Solid Edge part; units mm, degrees
sketch "Sketch1" plane through (0, 0, 0) normal (0, 0, 1) x (1, 0, 0)
  line L0 (-12, 10) -> (12, 10)
  line L1 (12, -10) -> (12, 10)
  line L2 (-12, -10) -> (12, -10)
  line L3 (-12, -10) -> (-12, 10)
  circle A0 centre (-7, 5) radius 2.2
  circle A1 centre (-7, -5) radius 2.2
  circle A2 centre (7, -5) radius 2.2
  circle A3 centre (7, 5) radius 2.2
extrude "Protrusion1" add sketch "Sketch1" against normal blind 6
Geometry: final body of the model. Coordinates: model frame, mm. Give positions to 0.01 mm unless a question says otherwise; leave off trailing zeros. Write each loop counter-clockwise with the first axis right and the second up, starting at its lowest first coordinate (ties: lowest second). Pieces come first, ordered by that corner, then holes.
1. Section query C-C, the plane z = -0.9. Return loops of the section in (x, y).
2. Draft query along Y for faces 1 (the cylindrical face through (-4.9, 5.66, -2.96)), 2 (the flat face through (0, 10, -3)), 3 (the flat face through (0, -10, -3)), 4 (the flat face through (12, 0, -3)). Return one class per face: released by +Y, released by -Y, zero draft, split by the parting line, or undercut.
3. Section query A-A, the plane y = -5. Return loops of the section in (x, z), then the cut area to 3 significant figures.
4. Section query B-B, the plane x = -7. Return loops of the section in (y, z), then the cut area to 3 significant figures.
5. Pin query (flat end, axial travel): P1, Ø5.5, axis at x = -7, y = 5, coming from the -Z side. Return the tip coordinate at first contact, or that it passes through.
6. Line query: probe 1 along Y at (x, z) = (7, -1.4); probe 2 along X at (y, z) = (-6.5, -1.75); probe 3 along X at (y, z) = (-3.75, -4.85). Output: solid intervals per line, ascending.
Computed:
1. outline: (-12, -10) - (12, -10) - (12, 10) - (-12, 10) - close; hole circle Ø4.4 at (-7, -5); hole circle Ø4.4 at (-7, 5); hole circle Ø4.4 at (7, -5); hole circle Ø4.4 at (7, 5)
2. face 1: undercut
2. face 2: released by +Y
2. face 3: released by -Y
2. face 4: zero draft
3. outline: (-12, -6) - (-9.2, -6) - (-9.2, 0) - (-12, 0) - close; (-4.8, -6) - (4.8, -6) - (4.8, 0) - (-4.8, 0) - close; (9.2, -6) - (12, -6) - (12, 0) - (9.2, 0) - close
3. area: 91.2 mm2
4. outline: (-10, -6) - (-7.2, -6) - (-7.2, 0) - (-10, 0) - close; (-2.8, -6) - (2.8, -6) - (2.8, 0) - (-2.8, 0) - close; (7.2, -6) - (10, -6) - (10, 0) - (7.2, 0) - close
4. area: 67.2 mm2
5. P1: stops at z = -6
6. probe 1: y = -10 to -7.2, -2.8 to 2.8, 7.2 to 10
6. probe 2: x = -12 to -8.61, -5.39 to 5.39, 8.61 to 12
6. probe 3: x = -12 to -8.81, -5.19 to 5.19, 8.81 to 12
